Source: CAD feature listing. Evaluate the final solid. Frame: model axes, mm. A direction names the side the tool comes from. Give positions to 0.01 mm unless a question says otherwise; leave off trailing zeros. Order: outer loops, then holes, each group sorted by start corner. A loop starts at its lowest first (then second) coordinate and runs counter-clockwise, first axis right, second up. Notation, with made-up numbers: M 64,23 L 90,23 A19 cw 90,37 Z; hole C -32.75,35.25 d1. An arc over 180 degrees is marked long. Return JSON: item names as keys, results as strings.
Autodesk Inventor part; units mm, degrees
ref_plane "YZ Plane" through (0, 0, 0) normal (1, 0, 0) x (0, 1, 0)
ref_plane "XZ Plane" through (0, 0, 0) normal (0, 1, 0) x (-1, 0, 0)
ref_plane "XY Plane" through (0, 0, 0) normal (0, 0, 1) x (1, 0, 0)
sketch "Sketch2" plane through (0, 0, 0) normal (0, 0, 1) x (1, 0, 0)
  circle A0 centre (0, 0) radius 9.5
  dimension "d0" = 19
extrude "Extrusion1" add sketch "Sketch2" along normal blind 11
sketch "Sketch5" plane through (0, 0, 11) normal (0, 0, 1) x (1, 0, 0)
  circle A0 centre (0, 0) radius 15
  dimension "d17" = 30
extrude "Extrusion4" add sketch "Sketch5" against normal blind 5
sketch "Sketch3" plane through (0, 0, 11) normal (0, 0, 1) x (1, 0, 0)
  circle A0 centre (0, -4) radius 1.75
  circle A1 centre (0, 4) radius 1.75
  line L0 (0, -9.5) -> (0, 9.5) construction
  circle A2 centre (0, 0) radius 9.5 construction
  dimension "d3" = 3.5
  dimension "d4" = 3.5
  dimension "d5" = 8
  dimension "d6" = 4
extrude "Extrusion2" cut sketch "Sketch3" against normal through all
sketch "Sketch4" plane through (0, 0, 11) normal (0, 0, 1) x (1, 0, 0)
  circle A0 centre (-10, 0) radius 2.1
  circle A1 centre (10, 0) radius 2.1
  line L0 (10, 0) -> (-10, 0) construction
  point P0 (0, 0)
  point P1 (0, 0)
  dimension "d9" = 4.2
  dimension "d10" = 4.2
  dimension "d11" = 20
extrude "Extrusion3" cut sketch "Sketch4" against normal blind 5
chamfer "Chamfer1" distance 0.5 angle 45 2 edges at (7.9, 0, 11) (-12.1, 0, 11)
equation "\"d5\" = 2 * d6"
properties part number "Motor Adapter"
1. Draft query along X for faces 1 (the face through (-14.985, 0.66, 8.535)), 2 (the face through (0, -10, 6)), 3 (the face through (-12.1, 0.09, 8.28)). Return one class per face: pulls with the +X half, pulls with the -X half, needs draft (parallel to the pull), parting line crosses it, or undercut.
Evaluation:
{"face 1": "parting line crosses it", "face 2": "needs draft", "face 3": "undercut"}
2. Section query D-D (x = -10). Return loops of the section in (y, z).
Evaluation:
{"outline": "M -11.18,6 L -2.1,6 L -2.1,10.5 L -2.6,11 L -11.18,11 Z; M 2.1,6 L 11.18,6 L 11.18,11 L 2.6,11 L 2.1,10.5 Z"}
3. Section query A-A (x = 0). Return loops of the section in (y, z), then the cut area to 3 significant figures.
Evaluation:
{"outline": "M -15,6 L -9.5,6 L -9.5,0 L -5.75,0 L -5.75,11 L -15,11 Z; M -2.25,0 L 2.25,0 L 2.25,11 L -2.25,11 Z; M 5.75,0 L 9.5,0 L 9.5,6 L 15,6 L 15,11 L 5.75,11 Z", "area": "187 mm^2"}
4. Set-up query: faces 4 (the face through (9, 0, 6)), 5 (the face through (-0.38, -5.71, 5.58)), 6 (the face through (4.38, 8.43, 2.96)). Return all of +Z, -Z, +X, -X, +Y, -Y with unobstructed straight access to the full face (end or side cutting, diameter ignored); none if empty.
Evaluation:
{"face 4": "+Z", "face 5": "+Z, -Z", "face 6": "-Z"}
5. First-contact query: pin 1 (5 mm diameter, centred on y = -5, z = 8.5, fed in from -X); pin 2 (2 mm diameter, centred on y = -9, z = 6.5, fed in from -X); pin 3 (6 mm diameter, centred on x = 4, z = 8, fed in from -Y). Flat tips, straight axial feed; report the tip coordinate or a pass-through.
Evaluation:
{"pin 1": "stops at x = -14.79", "pin 2": "stops at x = -12.69", "pin 3": "stops at y = -14.97"}
6. Section query B-B (y = 4). Return loops of the section in (x, z), then the cut area to 3 significant figures.
Evaluation:
{"outline": "M -14.46,6 L -8.62,6 L -8.62,0 L -1.75,0 L -1.75,11 L -14.46,11 Z; M 1.75,0 L 8.62,0 L 8.62,6 L 14.46,6 L 14.46,11 L 1.75,11 Z", "area": "209 mm^2"}
7. Section query C-C (z = 10). Return loops of the section in (x, y).
Evaluation:
{"outline": "C 0,0 d30; hole C -10,0 d4.2; hole C 0,-4 d3.5; hole C 0,4 d3.5; hole C 10,0 d4.2"}
8. Ray query, probe 1 along Y at (x, z) = (0, 5.75); probe 2 along Y at (x, z) = (0, 7.5); probe 3 along Z at (x, y) = (11.5, -9). Return the intervals inside material, ascending.
Evaluation:
{"probe 1": "y = -9.5 to -5.75, -2.25 to 2.25, 5.75 to 9.5", "probe 2": "y = -15 to -5.75, -2.25 to 2.25, 5.75 to 15", "probe 3": "z = 6 to 11"}
